Study the drawing (mm; zero at the part's minimum x, y, z) and answer. A direction names the side the tool comes from. Round coordinates to 2 decimals unless told otherwise and drop trailing zeros. Write each loop counter-clockwise with the first axis right and the second up, starting at its lowest first coordinate (ties: lowest second). Pieces come first, ordered by that corner, then holes. Notation, with made-up numbers: (79.5, 73) - (122.5, 73) arc R20 cw to (122.5, 106) - close; hole circle Ø1 at (80.25, 5.25). An arc over 180 degrees is marked (long way). Return JSON: item names as keys, results as strings. Group by question number.
(1) Which of the six approach directions +Z, -Z, +X, -X, +Y, -Y give full straight-line access (tool end or side, diameter ignored) to the marked faces 4 and 5?
(2) Section D-D, the plane z = 2.5 is taken. Write down the section's boundary in (x, y), then the cut area to 3 significant figures.
(3) Section B-B, the plane z = 10 is taken. Write down the section's boundary in (x, y).
(4) Find the intervals of material crossed by line 1 along Y through (x, z) = (11.5, 18.25); line 2 along X through (y, z) = (10, 1); line 3 along X through (y, z) = (9.8, 4.25), in increasing order. Write a range as [from, to].
(5) Determine the mould class of the marked faces 1, 2 and 3 for opening direction Y: +Y half, -Y half, draft (parallel to the pull), parting line (faces both ways), or undercut.
(6) Section A-A, the plane x = 10 is taken. Write down the section's boundary in (y, z).
(7) Section C-C, the plane y = 5.5 is taken. Write down the section's boundary in (x, z), then the cut area to 3 significant figures.
(8) Each of these flat-tipped pins is pushed along its axis until it touches: pin 1 (1 mm diameter, centred on x = 4.5, y = 8.5, fed in from +Z); pin 2 (1.8 mm diameter, centred on x = 11.5, y = 10.5, fed in from -Z); pin 3 (8 mm diameter, centred on y = 15.5, z = 15, fed in from +X). Where does it stop, or does it pass through?
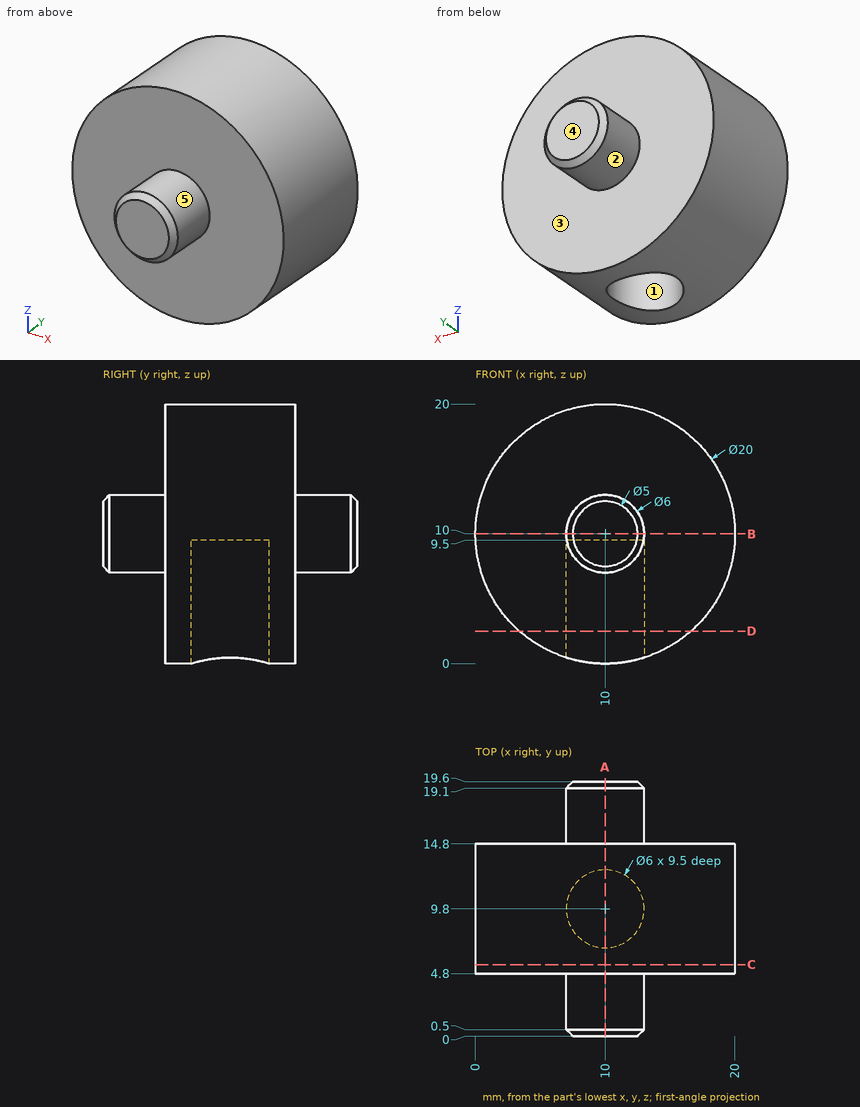
Working result:
{
 "1": {"face 4": "+Z, -Z, +X, -X, +Y", "face 5": "-Y"},
 "2": {"outline": "(3.39, 4.8) - (16.61, 4.8) - (16.61, 14.8) - (3.39, 14.8) - close; hole circle Ø6 at (10, 9.8)", "area": "104 mm^2"},
 "3": {"outline": "(0, 4.8) - (7, 4.8) - (7, 0.5) - (7.5, 0) - (12.5, 0) - (13, 0.5) - (13, 4.8) - (20, 4.8) - (20, 14.8) - (13, 14.8) - (13, 19.1) - (12.5, 19.6) - (7.5, 19.6) - (7, 19.1) - (7, 14.8) - (0, 14.8) - close"},
 "4": {"line 1": "y = [4.8, 14.8]", "line 2": "x = [5.64, 7.01], [12.99, 14.36]", "line 3": "x = [1.82, 7], [13, 18.18]"},
 "5": {"face 1": "undercut", "face 2": "draft", "face 3": "+Y half"},
 "6": {"outline": "(0, 7.5) - (0.5, 7) - (4.8, 7) - (4.8, 0) - (6.8, 0) - (6.8, 9.5) - (12.8, 9.5) - (12.8, 0) - (14.8, 0) - (14.8, 7) - (19.1, 7) - (19.6, 7.5) - (19.6, 12.5) - (19.1, 13) - (14.8, 13) - (14.8, 20) - (4.8, 20) - (4.8, 13) - (0.5, 13) - (0, 12.5) - close"},
 "7": {"outline": "circle Ø20 at (10, 10)", "area": "314 mm^2"},
 "8": {"pin 1": "stops at z = 18.66", "pin 2": "stops at z = 9.5", "pin 3": "stops at x = 19.94"}
}
